Study the drawing (mm; zero at the part's minimum x, y, z) and answer. Coordinates: 2 decimals unless noted, no trailing zeros. Order: outer loops, then holes, each group sorted by start corner. A loop starts at its lowest first (then second) coordinate and runs counter-clockwise, first axis right, second up.
1. The part is cut by section D-D, the plane x = 38.5. Give the vertices of the cut face in (y, z), then the cut area to 3 significant figures.
2. Determine the mould class of the marked faces 1 and 2 for opening direction Y: +Y half, -Y half, draft (parallel to the pull), parting line (faces both ways), or undercut.
3. The part is cut by section A-A, the plane x = 30.5. Give the vertices of the cut face in (y, z).
4. The part is cut by section B-B, the plane z = 2.35. Give the vertices of the cut face in (x, y).
5. Flat-ended cylindrical pins translate along their axes: pin 1 Ø2 at (x, y) = (40.5, 2.5) entering from -Z; pin 2 Ø1.5 at (x, y) = (37.5, 22) entering from +Z. Find the tip coordinate at first contact, or state that the pin passes through.
6. Find the intervals of material crossed by probe 1 along Y at (x, z) = (27, 2.4); probe 2 along Y at (x, z) = (40.5, 2.8); probe 3 along Y at (x, z) = (2.5, 4.25), in increasing order.
7. The part is cut by section C-C, the plane y = 13. Give the vertices of the cut face in (x, z), then the cut area to 3 significant figures.
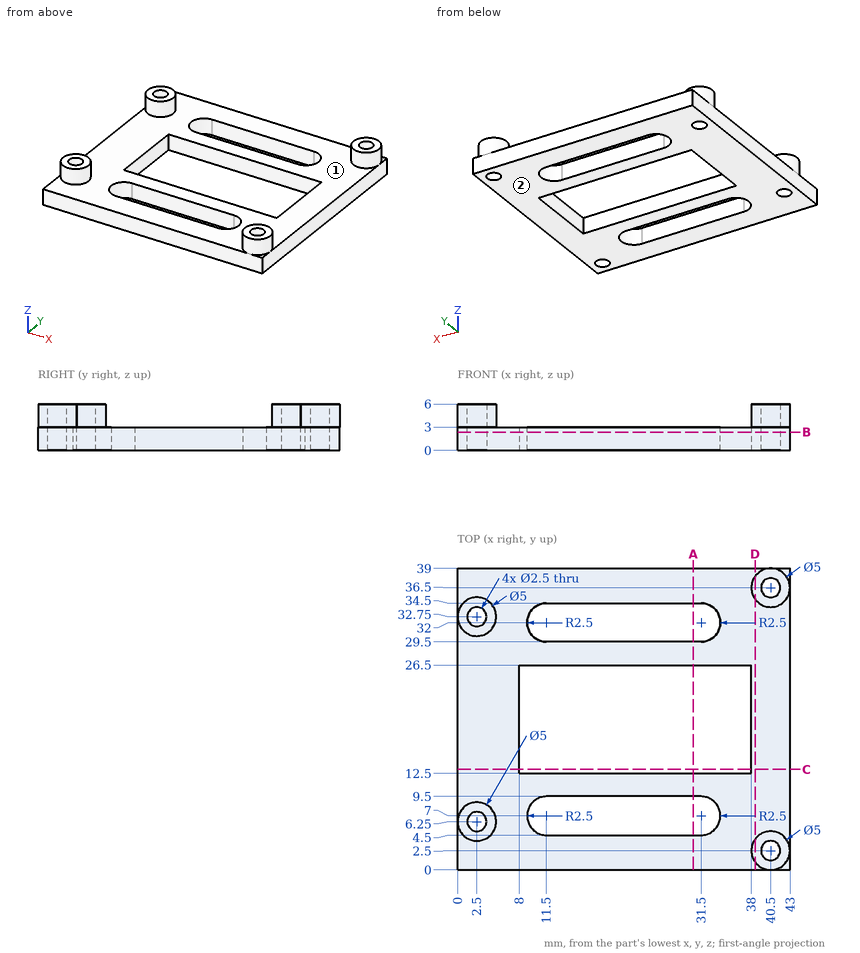
Geometry says:
1. outline: (0, 0) - (39, 0) - (39, 3) - (38, 3) - (38, 6) - (35, 6) - (35, 3) - (4, 3) - (4, 6) - (1, 6) - (1, 3) - (0, 3) - close
1. area: 135 mm2
2. face 1: undercut
2. face 2: draft
3. outline: (0, 0) - (4.5, 0) - (4.5, 3) - (0, 3) - close; (9.5, 0) - (12.5, 0) - (12.5, 3) - (9.5, 3) - close; (26.5, 0) - (29.5, 0) - (29.5, 3) - (26.5, 3) - close; (34.5, 0) - (39, 0) - (39, 3) - (34.5, 3) - close
4. outline: (0, 0) - (43, 0) - (43, 39) - (0, 39) - close; hole circle Ø2.5 at (2.5, 6.25); hole circle Ø2.5 at (2.5, 32.75); hole (8, 12.5) - (38, 12.5) - (38, 26.5) - (8, 26.5) - close; hole (11.5, 4.5) - (31.5, 4.5) arc R2.5 ccw to (31.5, 9.5) - (11.5, 9.5) arc R2.5 ccw to start; hole (11.5, 29.5) - (31.5, 29.5) arc R2.5 ccw to (31.5, 34.5) - (11.5, 34.5) arc R2.5 ccw to start; hole circle Ø2.5 at (40.5, 2.5); hole circle Ø2.5 at (40.5, 36.5)
5. pin 1: passes through
5. pin 2: stops at z = 3
6. probe 1: y = 0 to 4.5, 9.5 to 12.5, 26.5 to 29.5, 34.5 to 39
6. probe 2: y = 0 to 1.25, 3.75 to 35.25, 37.75 to 39
6. probe 3: y = 3.75 to 5, 7.5 to 8.75, 30.25 to 31.5, 34 to 35.25
7. outline: (0, 0) - (8, 0) - (8, 3) - (0, 3) - close; (38, 0) - (43, 0) - (43, 3) - (38, 3) - close
7. area: 39.0 mm2
